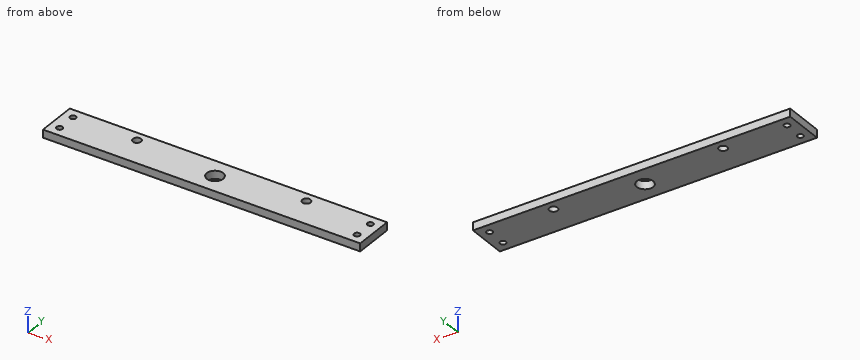
from build123d import *

# Parameters (mm, degrees)
SKETCH1_W           = 320
SKETCH1_H           = 40
BOSS_EXTRUDE1_DEPTH = 8
CUT_EXTRUDE1_REACH  = 10
SKETCH2_R           = 3
CUT_EXTRUDE2_REACH  = 10
SKETCH3_R           = 4.15
SKETCH3_R_2         = 8.25


with BuildPart() as part:
    # Sketch1 → Boss-Extrude1 (new body)
    with BuildSketch(Plane.XY):
        Rectangle(SKETCH1_W, SKETCH1_H)
    extrude(amount=BOSS_EXTRUDE1_DEPTH)

    # Sketch2 → Cut-Extrude1 (cut, up to next)
    with BuildSketch(Plane.XY.offset(8), mode=Mode.PRIVATE) as cut_extrude1_sk1:
        with Locations((-150, 10)):
            Circle(SKETCH2_R)
    cut_extrude1_tool1 = extrude(cut_extrude1_sk1.sketch, amount=-CUT_EXTRUDE1_REACH, mode=Mode.PRIVATE) & part.part
    add(cut_extrude1_tool1.solids().sort_by_distance((-150, 10, 8))[0], mode=Mode.SUBTRACT)
    # Sketch2 → Cut-Extrude1 (cut, up to next)
    with BuildSketch(Plane.XY.offset(8), mode=Mode.PRIVATE) as cut_extrude1_sk2:
        with Locations((-150, -10)):
            Circle(SKETCH2_R)
    cut_extrude1_tool2 = extrude(cut_extrude1_sk2.sketch, amount=-CUT_EXTRUDE1_REACH, mode=Mode.PRIVATE) & part.part
    add(cut_extrude1_tool2.solids().sort_by_distance((-150, -10, 8))[0], mode=Mode.SUBTRACT)
    # Sketch2 → Cut-Extrude1 (cut, up to next)
    with BuildSketch(Plane.XY.offset(8), mode=Mode.PRIVATE) as cut_extrude1_sk3:
        with Locations((150, -10)):
            Circle(SKETCH2_R)
    cut_extrude1_tool3 = extrude(cut_extrude1_sk3.sketch, amount=-CUT_EXTRUDE1_REACH, mode=Mode.PRIVATE) & part.part
    add(cut_extrude1_tool3.solids().sort_by_distance((150, -10, 8))[0], mode=Mode.SUBTRACT)
    # Sketch2 → Cut-Extrude1 (cut, up to next)
    with BuildSketch(Plane.XY.offset(8), mode=Mode.PRIVATE) as cut_extrude1_sk4:
        with Locations((150, 10)):
            Circle(SKETCH2_R)
    cut_extrude1_tool4 = extrude(cut_extrude1_sk4.sketch, amount=-CUT_EXTRUDE1_REACH, mode=Mode.PRIVATE) & part.part
    add(cut_extrude1_tool4.solids().sort_by_distance((150, 10, 8))[0], mode=Mode.SUBTRACT)

    # Sketch3 → Cut-Extrude2 (cut, up to next)
    with BuildSketch(Plane.XY.offset(8), mode=Mode.PRIVATE) as cut_extrude2_sk1:
        with Locations((-85.5, 10)):
            Circle(SKETCH3_R)
    cut_extrude2_tool1 = extrude(cut_extrude2_sk1.sketch, amount=-CUT_EXTRUDE2_REACH, mode=Mode.PRIVATE) & part.part
    add(cut_extrude2_tool1.solids().sort_by_distance((-85.5, 10, 8))[0], mode=Mode.SUBTRACT)
    # Sketch3 → Cut-Extrude2 (cut, up to next)
    with BuildSketch(Plane.XY.offset(8), mode=Mode.PRIVATE) as cut_extrude2_sk2:
        with Locations((85.5, 10)):
            Circle(SKETCH3_R)
    cut_extrude2_tool2 = extrude(cut_extrude2_sk2.sketch, amount=-CUT_EXTRUDE2_REACH, mode=Mode.PRIVATE) & part.part
    add(cut_extrude2_tool2.solids().sort_by_distance((85.5, 10, 8))[0], mode=Mode.SUBTRACT)
    # Sketch3 → Cut-Extrude2 (cut, up to next)
    with BuildSketch(Plane.XY.offset(8), mode=Mode.PRIVATE) as cut_extrude2_sk3:
        Circle(SKETCH3_R_2)
    cut_extrude2_tool3 = extrude(cut_extrude2_sk3.sketch, amount=-CUT_EXTRUDE2_REACH, mode=Mode.PRIVATE) & part.part
    add(cut_extrude2_tool3.solids().sort_by_distance((0, 0, 8))[0], mode=Mode.SUBTRACT)


solid = part.part
Part model, mm, in its own coordinate system. Coordinates: 2 decimals unless noted, no trailing zeros. Loops run counter-clockwise (first coordinate to the right, second up) from the corner with the lowest first, then second, coordinate; pieces in that order, holes last. Notation, with made-up numbers: (48, -8.5) -> (53, -8.5) arc R16 ccw to (53, 18.5) -> close; hole circle Ø7 at (89, -31). An arc over 180 degrees is marked (long way). Use a Markdown table: item, result. Add a question column.
Item 1: Flat gauge pins, fed straight in: P1, Ø5, axis at x = 150, y = -10, coming from the +Z side; P2, Ø13.5, axis at x = 85.5, y = 10, coming from the +Z side. Where does each tip first touch, or does it go through?
Item 2: Probe probe 1 along Y at (x, z) = (-150, 5.75); probe 2 along X at (y, z) = (9, 3.25); probe 3 along X at (y, z) = (8.5, 7.75). List the from-to ranges inside material, lowest first.
Item 3: Band-saw the part on C-C on x = 150. Write the cut outline in (y, z), plus the area to 3 significant figures.
Item 4: Band-saw the part on B-B on y = 0. Write the cut outline in (x, z), plus the area to 3 significant figures.
Item 5: Band-saw the part on A-A on x = 0. Write the cut outline in (y, z), plus the area to 3 significant figures.
Geometry says:
| question | item | result |
|---|---|---|
| 1 | P1 | through |
| 1 | P2 | z = 8 |
| 2 | probe 1 | -20 to -13, -7 to 7, 13 to 20 |
| 2 | probe 2 | -160 to -152.83, -147.17 to -89.53, -81.47 to 81.47, 89.53 to 147.17, 152.83 to 160 |
| 2 | probe 3 | -160 to -152.6, -147.4 to -89.37, -81.63 to 81.63, 89.37 to 147.4, 152.6 to 160 |
| 3 | outline | (-20, 0) -> (-13, 0) -> (-13, 8) -> (-20, 8) -> close; (-7, 0) -> (7, 0) -> (7, 8) -> (-7, 8) -> close; (13, 0) -> (20, 0) -> (20, 8) -> (13, 8) -> close |
| 3 | area | 224 mm² |
| 4 | outline | (-160, 0) -> (-8.25, 0) -> (-8.25, 8) -> (-160, 8) -> close; (8.25, 0) -> (160, 0) -> (160, 8) -> (8.25, 8) -> close |
| 4 | area | 2,430 mm² |
| 5 | outline | (-20, 0) -> (-8.25, 0) -> (-8.25, 8) -> (-20, 8) -> close; (8.25, 0) -> (20, 0) -> (20, 8) -> (8.25, 8) -> close |
| 5 | area | 188 mm² |
